Input: part model. Units: mm. Frame: model coordinates. A direction names the side the tool comes from. Round coordinates to 2 decimals unless told otherwise and drop trailing zeros. Loops run counter-clockwise (first coordinate to the right, second up) from the corner with the lowest first, then second, coordinate; pieces in that order, holes last. Notation, with made-up numbers: (52.25, -34) -> (106.25, -34) arc R23 cw to (106.25, 0) -> close; hole circle Ø5 at (86.25, 35.25). An arc over 180 degrees is marked (long way). Answer in a Markdown table with one row per item. Add a question column.
Q1. Reachability of faces 4 (the face through (54.62, -0.03, 42.29)), 5 (the face through (-32, 0, 70)), 6 (the face through (1, -91, 35)) from +Z, -Z, +X, -X, +Y, -Y: full face, straight path, thin tool, end or side. Return the list, or none.
Q2. Ray query, L1, parallel to Y at x = -93.5, z = 68; L2, parallel to X at y = 66.5, z = 55; L3, parallel to X at y = 83, z = 69. Return the intervals inside material, ascending. Write a range as from..to.
Q3. Section D-D, the plane z = 81.5. Output: boundary loops of the cut face in (x, y), and give its area (3 significant figures).
Q4. Pin query (flat end, axial travel): pin 1 (6 mm diameter, centred on x = -27, y = 96, fed in from +Z); pin 2 (4 mm diameter, centred on x = -45.5, z = 39.5, fed in from -Y); pin 3 (6 mm diameter, centred on y = 81, z = 21, fed in from +X). Return the tip coordinate at first contact, or that it passes through.
Q5. Mould query, pull axis X, two halves, no side actions, for faces 1 (the face through (-104.9, -107.22, 3.56)), 2 (the face through (-83.784, -85.631, 43.268)), 3 (the face through (44, -88, 0)). Classes: pulls with the +X half, pulls with the -X half, needs draft (parallel to the pull), parting line crosses it, or undercut.
Q6. Section A-A, the plane z = 17. Give the number of separate pieces and of enclosed holes in the cut face, and give its area (3 significant figures).
```python
from build123d import *

# Parameters (mm, degrees)
BOSS_EXTRUDE1_DEPTH = 70


with BuildPart() as part:
    # Sketch1 → Revolve1 (revolve)
    with BuildSketch(Plane(origin=(0, 0, 0), x_dir=(0, 0, -1), z_dir=(1, 0, 0)), mode=Mode.PRIVATE) as revolve1_sk:
        Polygon((0, 101.6), (-101.15, 0), (-96.916744498, 0), (0, 97.347911428), align=None)
    revolve(revolve1_sk.sketch.rotate(Axis((0, 0, 101.15), (0, 0, -1)), 270), axis=Axis((0, 0, 101.15), (0, 0, -1)))

    # Sketch3 → Boss-Extrude1 (add)
    with BuildSketch(Plane.XY):
        Polygon((-1, 1), (-150, 1), (-150, -1), (-1, -1), (-1, -150), (1, -150), (1, -1), (150, -1), (150, 1), (1, 1), (1, 150), (-1, 150), align=None)
    extrude(amount=BOSS_EXTRUDE1_DEPTH)

    # Sketch5 → Cut-Revolve1 (revolve, cut)
    with BuildSketch(Plane(origin=(0, 0, 0), x_dir=(0, 0, -1), z_dir=(1, 0, 0))):
        Polygon((-96.916744498, 0), (6.133899753, 103.041259066), (0, 0), align=None)
    revolve(axis=Axis((0, 0, 0), (0, 0, 1)), mode=Mode.SUBTRACT)

    # Sketch6 → Revolve2 (revolve)
    with BuildSketch(Plane(origin=(0, 0, 0), x_dir=(0, 0, -1), z_dir=(1, 0, 0))):
        Polygon((0, 150), (-70, 101.145056725), (-70, 106.195161711), (-7.235856299, 150), align=None)
    revolve(axis=Axis((0, 0, 106.204880544), (0, 0, -1)))

    # Sketch7 → Cut-Revolve2 (revolve, cut)
    with BuildSketch(Plane(origin=(0, 0, 0), x_dir=(0, 0, -1), z_dir=(1, 0, 0)), mode=Mode.PRIVATE) as cut_revolve2_sk:
        Polygon((-7.235856299, 149.99666663), (-70, 106.190453294), (-70, 150), (-70, 151.803393864), (-4.647235207, 151.803393864), align=None)
    revolve(cut_revolve2_sk.sketch.rotate(Axis((0, 0, 108.547255844), (0, 0, -1)), 269.618033807), axis=Axis((0, 0, 108.547255844), (0, 0, -1)), mode=Mode.SUBTRACT)


solid = part.part
```
Answer block:
| question | item | result |
|---|---|---|
| 1 | face 4 | -Z |
| 1 | face 5 | +Z |
| 1 | face 6 | none |
| 2 | L1 | -53.22..-42.1, -1..1, 42.1..53.22 |
| 2 | L2 | -95.85..-89.64, -1..1, 89.64..95.85 |
| 2 | L3 | -67.35..-59.02, -1..1, 59.02..67.35 |
| 3 | outline | circle Ø39.47 at (0, 0); hole circle Ø30.97 at (0, 0) |
| 3 | area | 471 mm^2 |
| 4 | pin 1 | z = 70 |
| 4 | pin 2 | y = -120.75 |
| 4 | pin 3 | x = 117.94 |
| 5 | face 1 | pulls with the -X half |
| 5 | face 2 | undercut |
| 5 | face 3 | needs draft |
| 6 | separate pieces | 1 |
| 6 | enclosed holes | 5 |
| 6 | area | 7,090 mm^2 |
